Design review of the part built by this model. Coordinates are the model's own, in mm. Face numbers are marked on the shaded views. A direction names the side the tool comes from. Round coordinates to 2 decimals unless told otherwise and drop trailing zeros. Write each loop counter-clockwise with the first axis right and the second up, starting at its lowest first coordinate (ties: lowest second). Pieces come first, ordered by that corner, then holes. Notation, with made-up numbers: (38, 56) -> (93, 56) arc R14 cw to (93, 66) -> close; hole circle Ø3 at (51, 87). An arc over 180 degrees is marked (long way). One line per question, with ' | ' between items. Start each with the question number.
1) Consider section D-D (z = 0.5). Give the boundary of the cut face in (x, y), then the cut area to 3 significant figures.
2) Consider section B-B (y = 1.5). Count the separate pieces of the cut face and the enclosed holes in it, then the cut area to 3 significant figures.
3) Insertion check: pin 1 Ø8 at (x, z) = (-14.5, 14) entering from +Y; pin 2 Ø11.5 at (x, z) = (-13, -15.25) entering from +Y; pin 3 Ø1.2 at (y, z) = (-1.5, -7) entering from -X. Each pin has a flat end and moves straight along its axis. Give the tip position at first contact, or say it passes through.
4) Mouldability with a two-part tool opening along X and no side actions: class the marked faces 1, 2 and 3 as +X half, -X half, draft (parallel to the pull), parting line (faces both ways), or undercut.
5) Consider section A-A (x = 24). Give the boundary of the cut face in (y, z) (3 decimals).
6) For the marked faces 4, 5 and 6, list the 3-axis set-ups (+Z, -Z, +X, -X, +Y, -Y) from which the entire face can be reached by the end or side of a thin tool; tool diameter is ignored.
7) For probe 1 along X at (y, z) = (4.9, 15.25); probe 2 along X at (y, z) = (1, 15.25); probe 3 along Z at (x, y) = (-13, -0.75), list the stretches that pass through material, from the lowest coordinate up.
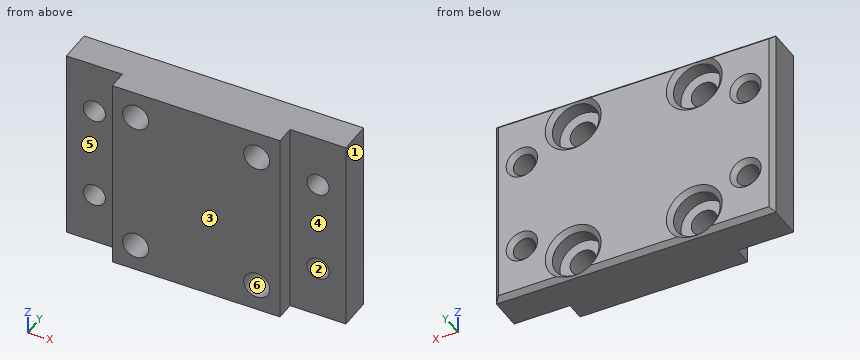
```python
from build123d import *

# Parameters (mm, degrees)
ESBO_O1_W                = 60
ESBO_O1_H                = 42
ESBO_O1_R                = 2.8
ESBO_O1_R_2              = 2.375
RESSALTO_EXTRUS_O1_DEPTH = 8
CORTE_EXTRUS_O1_START    = 8
ESBO_O1_3_R              = 5
CORTE_EXTRUS_O1_DEPTH    = 4
RESSALTO_EXTRUS_O4_START = -4
ESBO_O1_5_W              = 36
ESBO_O1_5_H              = 42
ESBO_O1_5_R              = 2.8
RESSALTO_EXTRUS_O4_DEPTH = 4
CHANFRO1_SIZE            = 1


with BuildPart() as part:
    # Esboço1 → Ressalto-extrusão1 (new body)
    with BuildSketch(Plane(origin=(0, 0, 0), x_dir=(1, 0, 0), z_dir=(0, 1, 0))):
        Rectangle(ESBO_O1_W, ESBO_O1_H)
        with Locations(Location((-13, 15.25, 0), (0, 0, 270))):
            Circle(ESBO_O1_R, mode=Mode.SUBTRACT)
        with Locations(Location((-13, -15.25, 0), (0, 0, 270))):
            Circle(ESBO_O1_R, mode=Mode.SUBTRACT)
        with Locations(Location((13, 15.25, 0), (0, 0, 270))):
            Circle(ESBO_O1_R, mode=Mode.SUBTRACT)
        with Locations(Location((13, -15.25, 0), (0, 0, 270))):
            Circle(ESBO_O1_R, mode=Mode.SUBTRACT)
        with Locations(Location((-24, 10, 0), (0, 0, 270))):
            Circle(ESBO_O1_R_2, mode=Mode.SUBTRACT)
        with Locations(Location((-24, -10, 0), (0, 0, 270))):
            Circle(ESBO_O1_R_2, mode=Mode.SUBTRACT)
        with Locations(Location((24, -10, 0), (0, 0, 270))):
            Circle(ESBO_O1_R_2, mode=Mode.SUBTRACT)
        with Locations(Location((24, 10, 0), (0, 0, 270))):
            Circle(ESBO_O1_R_2, mode=Mode.SUBTRACT)
    extrude(amount=RESSALTO_EXTRUS_O1_DEPTH)

    # Esboço1<3> → Corte-extrusão1 (cut)
    with BuildSketch(Plane(origin=(0, 0, 0), x_dir=(1, 0, 0), z_dir=(0, 1, 0)).offset(CORTE_EXTRUS_O1_START)):
        with Locations(Location((-13, 15.25, 0), (0, 0, 270))):
            Circle(ESBO_O1_3_R)
        with Locations(Location((13, 15.25, 0), (0, 0, 270))):
            Circle(ESBO_O1_3_R)
        with Locations(Location((13, -15.25, 0), (0, 0, 270))):
            Circle(ESBO_O1_3_R)
        with Locations(Location((-13, -15.25, 0), (0, 0, 270))):
            Circle(ESBO_O1_3_R)
    extrude(amount=-CORTE_EXTRUS_O1_DEPTH, mode=Mode.SUBTRACT)

    # Esboço1<5> → Ressalto-extrusão4 (add)
    with BuildSketch(Plane(origin=(0, 0, 0), x_dir=(1, 0, 0), z_dir=(0, 1, 0)).offset(RESSALTO_EXTRUS_O4_START)):
        Rectangle(ESBO_O1_5_W, ESBO_O1_5_H)
        with Locations(Location((13, -15.25, 0), (0, 0, 270))):
            Circle(ESBO_O1_5_R, mode=Mode.SUBTRACT)
        with Locations(Location((-13, -15.25, 0), (0, 0, 270))):
            Circle(ESBO_O1_5_R, mode=Mode.SUBTRACT)
        with Locations(Location((13, 15.25, 0), (0, 0, 270))):
            Circle(ESBO_O1_5_R, mode=Mode.SUBTRACT)
        with Locations(Location((-13, 15.25, 0), (0, 0, 270))):
            Circle(ESBO_O1_5_R, mode=Mode.SUBTRACT)
    extrude(amount=RESSALTO_EXTRUS_O4_DEPTH)

    # Chanfro1
    # the kernel refuses this chamfer: 1 mm, written as the material it takes off along each edge
    with BuildSketch(Plane(origin=(-30, 8, -23.571682988), x_dir=(0.9996219169112968, 0.027495876610585647, 0), z_dir=(0, 0, 1))) as chanfro1_piece_1:
        Polygon((CHANFRO1_SIZE * 0.999621916911, -CHANFRO1_SIZE * 0.0274958766106), (-CHANFRO1_SIZE * 0.0274958766106, -CHANFRO1_SIZE * 0.999621916911), (0, 0), align=None)
    extrude(amount=47.143365976, mode=Mode.SUBTRACT)
    with BuildSketch(Plane(origin=(-32.571682988, 8, 21), x_dir=(0, -0.9996219169112968, 0.027495876610585623), z_dir=(1, 0, 0)), Plane(origin=(32.571682988, 8, -21), x_dir=(0, -0.9996219169112968, -0.027495876610585623), z_dir=(-1, 0, 0))) as chanfro1_piece_2:
        Polygon((CHANFRO1_SIZE * 0.999621916911, CHANFRO1_SIZE * 0.0274958766106), (-CHANFRO1_SIZE * 0.0274958766106, CHANFRO1_SIZE * 0.999621916911), (0, 0), align=None)
    extrude(amount=65.143365976, mode=Mode.SUBTRACT)
    with BuildSketch(Plane(origin=(30, 8, 23.571682988), x_dir=(0.027495876610585623, -0.9996219169112968, 0), z_dir=(0, 0, -1))) as chanfro1_piece_3:
        Polygon((CHANFRO1_SIZE * 0.999621916911, CHANFRO1_SIZE * 0.0274958766106), (-CHANFRO1_SIZE * 0.0274958766106, CHANFRO1_SIZE * 0.999621916911), (0, 0), align=None)
    extrude(amount=47.143365976, mode=Mode.SUBTRACT)
    with BuildSketch(Plane(origin=(-24, 8, 10), x_dir=(0, 0, 1), z_dir=(-1, 0, 0))) as chanfro1_piece_4:
        Polygon((2.375, -CHANFRO1_SIZE), (2.375 + CHANFRO1_SIZE, 0), (2.375, 0), align=None)
    revolve(axis=Axis((-24, 8, 10), (0, 1, 0)), mode=Mode.SUBTRACT)
    with BuildSketch(Plane(origin=(-24, 8, -10), x_dir=(0, 0, 1), z_dir=(-1, 0, 0))) as chanfro1_piece_5:
        Polygon((2.375, -CHANFRO1_SIZE), (2.375 + CHANFRO1_SIZE, 0), (2.375, 0), align=None)
    revolve(axis=Axis((-24, 8, -10), (0, 1, 0)), mode=Mode.SUBTRACT)
    with BuildSketch(Plane(origin=(-13, 8, -15.25), x_dir=(0, 0, 1), z_dir=(-1, 0, 0))) as chanfro1_piece_6:
        Polygon((5, -CHANFRO1_SIZE), (5 + CHANFRO1_SIZE, 0), (5, 0), align=None)
    revolve(axis=Axis((-13, 8, -15.25), (0, 1, 0)), mode=Mode.SUBTRACT)
    with BuildSketch(Plane(origin=(24, 8, -10), x_dir=(0, 0, 1), z_dir=(-1, 0, 0))) as chanfro1_piece_7:
        Polygon((2.375, -CHANFRO1_SIZE), (2.375 + CHANFRO1_SIZE, 0), (2.375, 0), align=None)
    revolve(axis=Axis((24, 8, -10), (0, 1, 0)), mode=Mode.SUBTRACT)
    with BuildSketch(Plane(origin=(24, 8, 10), x_dir=(0, 0, 1), z_dir=(-1, 0, 0))) as chanfro1_piece_8:
        Polygon((2.375, -CHANFRO1_SIZE), (2.375 + CHANFRO1_SIZE, 0), (2.375, 0), align=None)
    revolve(axis=Axis((24, 8, 10), (0, 1, 0)), mode=Mode.SUBTRACT)
    with BuildSketch(Plane(origin=(13, 8, -15.25), x_dir=(0, 0, 1), z_dir=(-1, 0, 0))) as chanfro1_piece_9:
        Polygon((5, -CHANFRO1_SIZE), (5 + CHANFRO1_SIZE, 0), (5, 0), align=None)
    revolve(axis=Axis((13, 8, -15.25), (0, 1, 0)), mode=Mode.SUBTRACT)
    with BuildSketch(Plane(origin=(-13, 8, 15.25), x_dir=(0, 0, 1), z_dir=(-1, 0, 0))) as chanfro1_piece_10:
        Polygon((5, -CHANFRO1_SIZE), (5 + CHANFRO1_SIZE, 0), (5, 0), align=None)
    revolve(axis=Axis((-13, 8, 15.25), (0, 1, 0)), mode=Mode.SUBTRACT)
    with BuildSketch(Plane(origin=(13, 8, 15.25), x_dir=(0, 0, 1), z_dir=(-1, 0, 0))) as chanfro1_piece_11:
        Polygon((5, -CHANFRO1_SIZE), (5 + CHANFRO1_SIZE, 0), (5, 0), align=None)
    revolve(axis=Axis((13, 8, 15.25), (0, 1, 0)), mode=Mode.SUBTRACT)


solid = part.part
```
From the geometry:
1) outline: (-30, 0) -> (-18, 0) -> (-18, -4) -> (18, -4) -> (18, 0) -> (30, 0) -> (30, 7) -> (29, 8) -> (-29, 8) -> (-30, 7) -> close | area: 623 mm2
2) separate pieces: 1 | enclosed holes: 8 | area: 2,350 mm2
3) pin 1: stops at y = 7.95 | pin 2: stops at y = 7.75 | pin 3: stops at x = -18
4) face 1: +X half | face 2: undercut | face 3: draft
5) outline: (0, -21) -> (7, -21) -> (8, -20) -> (8, -13.375) -> (7, -12.375) -> (0, -12.375) -> close; (0, -7.625) -> (7, -7.625) -> (8, -6.625) -> (8, 6.625) -> (7, 7.625) -> (0, 7.625) -> close; (0, 12.375) -> (7, 12.375) -> (8, 13.375) -> (8, 20) -> (7, 21) -> (0, 21) -> close
6) face 4: +Z, -Z, +X, -Y | face 5: +Z, -Z, -X, -Y | face 6: +Y, -Y
7) probe 1: x = -30 to -18, -8 to 8, 18 to 30 | probe 2: x = -30 to -15.8, -10.2 to 10.2, 15.8 to 30 | probe 3: z = -21 to -18.05, -12.45 to 12.45, 18.05 to 21
